```python
from build123d import *

# Parameters (mm, degrees)
BOSS_EXTRUDE1_DEPTH = 2.5
SKETCH4_W           = 2.2
SKETCH4_H           = 12.2
CUT_EXTRUDE1_DEPTH  = 159.133646009
CUT_EXTRUDE2_DEPTH  = 159.133646009


with BuildPart() as part:
    # Sketch1 → Boss-Extrude1 (new body)
    with BuildSketch(Plane.YZ):
        Polygon((50, 0), (50, 50), (35, 50), (35, 150), (-35, 150), (-35, 50), (-50, 50), (-50, 0), (0, 0), align=None)
    extrude(amount=BOSS_EXTRUDE1_DEPTH)

    # Sketch4 → Cut-Extrude1 (cut, through all)
    with BuildSketch(Plane(origin=(0, 0, 0), x_dir=(0, -1, 0), z_dir=(-1, 0, 0))):
        with Locations((-30, 32)):
            Rectangle(SKETCH4_W, SKETCH4_H)
        with Locations((30, 32)):
            Rectangle(SKETCH4_W, SKETCH4_H)
    extrude(amount=-CUT_EXTRUDE1_DEPTH, mode=Mode.SUBTRACT)

    # Sketch6 → Cut-Extrude2 (cut, through all)
    with BuildSketch(Plane(origin=(0, 0, 0), x_dir=(0, -1, 0), z_dir=(-1, 0, 0))):
        with BuildLine():
            Line((-25, 92.5), (-15, 92.5))
            ThreePointArc((-15, 92.5), (-12.5, 90), (-15, 87.5))
            Line((-15, 87.5), (-25, 87.5))
            ThreePointArc((-25, 87.5), (-27.5, 90), (-25, 92.5))
        make_face()
        with BuildLine():
            Line((15, 92.5), (25, 92.5))
            ThreePointArc((25, 92.5), (27.5, 90), (25, 87.5))
            Line((25, 87.5), (15, 87.5))
            ThreePointArc((15, 87.5), (12.5, 90), (15, 92.5))
        make_face()
    extrude(amount=-CUT_EXTRUDE2_DEPTH, mode=Mode.SUBTRACT)


solid = part.part
```
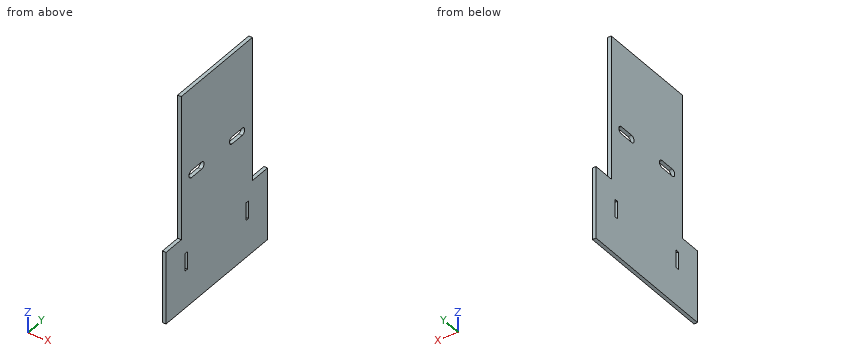
Source: CAD feature listing. Evaluate the final solid. Frame: model axes, mm. Round coordinates to 2 decimals unless told otherwise and drop trailing zeros. Loops run counter-clockwise (first coordinate to the right, second up) from the corner with the lowest first, then second, coordinate; pieces in that order, holes last. Notation, with made-up numbers: M 28,1 L 49,1 A34 ccw 49,33 Z; hole C -20,-3 d10. An arc over 180 degrees is marked long. Use a Markdown table: item, result. Add a question column.
1. Cut plane D-D, the plane z = 33. Output: boundary loops of the cut face in (x, y), and give its area (3 significant figures).
2. Cut plane C-C, the plane x = 1.3. Output: boundary loops of the cut face in (y, z).
3. Contact query for flat-ended pins moving along their axis: pin 1 (1.2 mm diameter, centred on x = 1.5, y = -41.5, fed in from +Z); pin 2 (0.8 mm diameter, centred on x = 1.5, z = 121.5, fed in from -Y). Output: stop coordinate, or through.
4. Ray query, line 1 along Y through (x, z) = (1.2, 28); line 2 along Z through (x, y) = (1.85, -18); line 3 along Y through (x, z) = (1.45, 90). Return the intervals inside material, ascending. Write a range as [from, to].
5. Cut plane B-B, the plane z = 90. Output: boundary loops of the cut face in (x, y).
6. Cut plane A-A, the plane y = 21.5. Output: boundary loops of the cut face in (x, z), and give its area (4 significant figures).
Solution:
| question | item | result |
|---|---|---|
| 1 | outline | M 0,-50 L 2.5,-50 L 2.5,-31.1 L 0,-31.1 Z; M 0,-28.9 L 2.5,-28.9 L 2.5,28.9 L 0,28.9 Z; M 0,31.1 L 2.5,31.1 L 2.5,50 L 0,50 Z |
| 1 | area | 239 mm2 |
| 2 | outline | M -50,0 L 50,0 L 50,50 L 35,50 L 35,150 L -35,150 L -35,50 L -50,50 Z; hole M -31.1,25.9 L -28.9,25.9 L -28.9,38.1 L -31.1,38.1 Z; hole M -25,87.5 L -15,87.5 A2.5 ccw -15,92.5 L -25,92.5 A2.5 ccw Z; hole M 15,87.5 L 25,87.5 A2.5 ccw 25,92.5 L 15,92.5 A2.5 ccw Z; hole M 28.9,25.9 L 31.1,25.9 L 31.1,38.1 L 28.9,38.1 Z |
| 3 | pin 1 | stops at z = 50 |
| 3 | pin 2 | stops at y = -35 |
| 4 | line 1 | y = [-50, -31.1], [-28.9, 28.9], [31.1, 50] |
| 4 | line 2 | z = [0, 87.5], [92.5, 150] |
| 4 | line 3 | y = [-35, -27.5], [-12.5, 12.5], [27.5, 35] |
| 5 | outline | M 0,-35 L 2.5,-35 L 2.5,-27.5 L 0,-27.5 Z; M 0,-12.5 L 2.5,-12.5 L 2.5,12.5 L 0,12.5 Z; M 0,27.5 L 2.5,27.5 L 2.5,35 L 0,35 Z |
| 6 | outline | M 0,0 L 2.5,0 L 2.5,87.5 L 0,87.5 Z; M 0,92.5 L 2.5,92.5 L 2.5,150 L 0,150 Z |
| 6 | area | 362.5 mm2 |
